from build123d import *

# Parameters (mm, degrees)
ESQUISSE1_W             = 12
ESQUISSE1_H             = 24
BOSS_EXTRU_1_DEPTH      = 6
ESQUISSE3_R             = 3.25
ENL_V_MAT_EXTRU_1_DEPTH = 10
ESQUISSE2_R             = 3.9
ENL_V_MAT_EXTRU_2_DEPTH = 10
ESQUISSE5_R             = 1.4
ENL_V_MAT_EXTRU_3_DEPTH = 22
ESQUISSE6_R             = 4.5
ESQUISSE6_R_2           = 3.25
BOSS_EXTRU_4_DEPTH      = 0.1
ESQUISSE8_W             = 21.223716878
ESQUISSE8_H             = 12.113313322
ENL_V_MAT_EXTRU_4_DEPTH = 19
ESQUISSE9_R             = 1.625
ENL_V_MAT_EXTRU_5_DEPTH = 19
ESQUISSE4_R             = 5
ESQUISSE4_R_2           = 3.25
BOSS_EXTRU_5_DEPTH      = 11
ESQUISSE11_W            = 12
ESQUISSE11_H            = 11.243517906
ESQUISSE11_R            = 3.25
BOSS_EXTRU_6_DEPTH      = 2.2
BOSS_EXTRU_6_DEPTH_BACK = 17
ESQUISSE12_W            = 21.1
ESQUISSE12_H            = 2
ENL_V_MAT_EXTRU_6_DEPTH = 13.1


with BuildPart() as part:
    # Esquisse1 → Boss.-Extru.1 (new body)
    with BuildSketch(Plane.XY):
        Rectangle(ESQUISSE1_W, ESQUISSE1_H)
    extrude(amount=BOSS_EXTRU_1_DEPTH)

    # Esquisse3 → Enlèv. mat.-Extru.1 (cut)
    with BuildSketch(Plane.XY.offset(6)):
        with Locations((0, 6)):
            Circle(ESQUISSE3_R)
    extrude(amount=-ENL_V_MAT_EXTRU_1_DEPTH, mode=Mode.SUBTRACT)

    # Esquisse2 → Enlèv. mat.-Extru.2 (cut)
    with BuildSketch(Plane.XY.offset(6)):
        with Locations((0, -6)):
            Circle(ESQUISSE2_R)
    extrude(amount=-ENL_V_MAT_EXTRU_2_DEPTH, mode=Mode.SUBTRACT)

    # Esquisse5 → Enlèv. mat.-Extru.3 (cut)
    with BuildSketch(Plane(origin=(6, 0, 0), x_dir=(0, 0, -1), z_dir=(1, 0, 0))):
        with Locations((-3, -6)):
            Circle(ESQUISSE5_R)
    extrude(amount=-ENL_V_MAT_EXTRU_3_DEPTH, mode=Mode.SUBTRACT)

    # Esquisse6 → Boss.-Extru.4 (add)
    with BuildSketch(Plane(origin=(0, 0, 0), x_dir=(-1, 0, 0), z_dir=(0, 0, -1))):
        with Locations((0, 6)):
            Circle(ESQUISSE6_R)
        with Locations(Location((0, 6, 0), (0, 0, 180))):
            Circle(ESQUISSE6_R_2, mode=Mode.SUBTRACT)
    extrude(amount=BOSS_EXTRU_4_DEPTH)

    # Esquisse7 → Révolution1 (revolve)
    with BuildSketch(Plane(origin=(0, 0, 0), x_dir=(0, 0, -1), z_dir=(1, 0, 0)), mode=Mode.PRIVATE) as r_volution1_sk:
        with BuildLine():
            Line((0.1, 10.5), (0.1, 9.25))
            ThreePointArc((0.1, 9.25), (2.398097039, 8.298097039), (3.35, 6))
            Line((3.35, 6), (4.6, 6))
            ThreePointArc((4.6, 6), (3.281980515, 9.181980515), (0.1, 10.5))
        make_face()
    revolve(r_volution1_sk.sketch.rotate(Axis((0, 6, -0.1), (0, 0, -1)), 90), axis=Axis((0, 6, -0.1), (0, 0, -1)))

    # Esquisse8 → Enlèv. mat.-Extru.4 (cut)
    with BuildSketch(Plane(origin=(6, 0, 0), x_dir=(0, 0, -1), z_dir=(1, 0, 0))):
        with Locations((12.811858439, 6.195094528)):
            Rectangle(ESQUISSE8_W, ESQUISSE8_H)
    extrude(amount=-ENL_V_MAT_EXTRU_4_DEPTH, mode=Mode.SUBTRACT)

    # Esquisse9 → Enlèv. mat.-Extru.5 (cut)
    with BuildSketch(Plane(origin=(6, 0, 0), x_dir=(0, 0, -1), z_dir=(1, 0, 0))):
        with Locations((-3, 6)):
            Circle(ESQUISSE9_R)
    extrude(amount=-ENL_V_MAT_EXTRU_5_DEPTH, mode=Mode.SUBTRACT)

    # Esquisse4 → Boss.-Extru.5 (add)
    with BuildSketch(Plane.XY.offset(6)):
        with Locations(Location((0, 6, 0), (0, 0, 180))):
            Circle(ESQUISSE4_R)
        with Locations((0, 6)):
            Circle(ESQUISSE4_R_2, mode=Mode.SUBTRACT)
    extrude(amount=BOSS_EXTRU_5_DEPTH)

    # Esquisse11 → Boss.-Extru.6 (add, two sides)
    with BuildSketch(Plane(origin=(0, 0, 0), x_dir=(-1, 0, 0), z_dir=(0, 0, -1))) as boss_extru_6_sk:
        with Locations((0, 6.378241047)):
            Rectangle(ESQUISSE11_W, ESQUISSE11_H)
        with Locations(Location((0, 6, 0), (0, 0, 180))):
            Circle(ESQUISSE11_R, mode=Mode.SUBTRACT)
    extrude(amount=BOSS_EXTRU_6_DEPTH)
    extrude(boss_extru_6_sk.sketch, amount=-BOSS_EXTRU_6_DEPTH_BACK)

    # Esquisse12 → Enlèv. mat.-Extru.6 (cut)
    with BuildSketch(Plane.ZY.offset(6)):
        with Locations((6.45, 11)):
            Rectangle(ESQUISSE12_W, ESQUISSE12_H)
    extrude(amount=-ENL_V_MAT_EXTRU_6_DEPTH, mode=Mode.SUBTRACT)


solid = part.part
Verification items for the finished model (mm, model axes). A direction names the side the tool comes from. Coordinates: 2 decimals unless noted, no trailing zeros. Write each loop counter-clockwise with the first axis right and the second up, starting at its lowest first coordinate (ties: lowest second). Pieces come first, ordered by that corner, then holes. Notation, with made-up numbers: (58.5, 28) -> (79.5, 28) arc R33 cw to (79.5, 59) -> close; hole circle Ø1 at (36, 24.5). An arc over 180 degrees is marked (long way). One line per item, written item: value. Start each with the question number.
Q1. Mould release check, pull along Y, two halves, no side actions. Record for faces 4 (the cylindrical face through (-4.8, -6.54, 1.71)), 5 (the flat face through (0, 10, 7)), 6 (the flat face through (0, 2, 17)), 7 (the flat face through (0, -12, 3)): pulls with the +Y half, pulls with the -Y half, needs draft (parallel to the pull), parting line crosses it, or undercut.
Q2. Cross-section at C-C on x = -2. Enter the section's corners in (y, z), and give its area (3 significant figures).
Q3. Go/stop test with flat-tipped pins: P1, Ø1.8, axis at x = -1, z = -1.5, coming from the -Y side; P2, Ø6, axis at x = 4.5, y = -9.5, coming from the +Z side; P3, Ø3.5, axis at x = 0.5, y = -4, coming from the -Z side. Record where each tip stops, or that it passes through.
Q4. Cross-section at B-B on y = -6. Enter the section's corners in (x, z), and give its area (3 significant figures).
Q5. Cross-section at A-A on z = 3. Enter the section's corners in (x, y) (3 decimals), and give its area (3 significant figures).
Q6. Thickness scan on L1, parallel to Y at x = 0, z = 3.75; L2, parallel to X at y = 6, z = 3.5; L3, parallel to Y at x = 0, z = 6.25. Record the ranges inside material, lowest first. Write a range as from..to.
Q7. Cross-section at D-D on z = 5.5. Enter the section's corners in (x, y), and give its area (3 significant figures).
Q8. Access from +Z, -Z, +X, -X, +Y, -Y to the whole of each face (thin tool, end or side, straight path). Record for faces 1 (the flat face through (6, 1, 5)), 2 (the flat face through (0, 0.756, -1)), 3 (the flat face through (3, -3, 6)).
Checked values:
1. face 4: undercut
1. face 5: pulls with the +Y half
1. face 6: needs draft
1. face 7: pulls with the -Y half
2. outline: (-12, 0) -> (-9.35, 0) -> (-9.35, 6) -> (-12, 6) -> close; (-2.65, 0) -> (0.76, 0) -> (0.76, -2.2) -> (4.53, -2.2) arc R2.56 cw to (3.44, -0.1) -> (3.44, 17) -> (0.76, 17) -> (0.76, 6) -> (-2.65, 6) -> close; (7.47, -2.2) -> (10, -2.2) -> (10, 17) -> (8.56, 17) -> (8.56, -0.1) arc R2.56 cw to start
2. area: 117 mm²
3. P1: stops at y = 0.76
3. P2: stops at z = 6
3. P3: passes through
4. outline: (-6, 0) -> (-3.9, 0) -> (-3.9, 1.6) -> (-6, 1.6) -> close; (-6, 4.4) -> (-3.9, 4.4) -> (-3.9, 6) -> (-6, 6) -> close; (3.9, 0) -> (6, 0) -> (6, 1.6) -> (3.9, 1.6) -> close; (3.9, 4.4) -> (6, 4.4) -> (6, 6) -> (3.9, 6) -> close
4. area: 13.4 mm²
5. outline: (-6, -12) -> (6, -12) -> (6, -7.4) -> (3.64, -7.4) arc R3.9 cw to (-3.64, -7.4) -> (-6, -7.4) -> close; (-6, -4.6) -> (-3.64, -4.6) arc R3.9 cw to (3.64, -4.6) -> (6, -4.6) -> (6, 10) -> (-6, 10) -> close; hole circle Ø6.5 at (0, 6)
5. area: 171 mm²
6. L1: y = -12..-9.9, -2.1..2.75, 9.25..10
6. L2: x = -6..-3.25, 3.25..6
6. L3: y = 0.76..2.75, 9.25..10
7. outline: (-6, -12) -> (6, -12) -> (6, 10) -> (-6, 10) -> close; hole circle Ø7.8 at (0, -6); hole circle Ø6.5 at (0, 6)
7. area: 183 mm²
8. face 1: +Z, -Z, +X, +Y, -Y
8. face 2: -Z, +X, -X, -Y
8. face 3: +Z, +X, -X, -Y
